Part model, mm, in its own coordinate system. Coordinates: 2 decimals unless noted, no trailing zeros. Loops run counter-clockwise (first coordinate to the right, second up) from the corner with the lowest first, then second, coordinate; pieces in that order, holes last. Notation, with made-up numbers: (52.25, 57) - (82.25, 57) arc R19 ccw to (82.25, 72) - close; hole circle Ø10 at (-14.75, 18.5). An arc over 180 degrees is marked (long way). Use a Markdown table: item, result. Add a question column.
1. Band-saw the part on C-C, the plane x = -0.75. Give the cut face in (y, z).
2. Drop flat-ended pins along their axis: pin 1 (1 mm diameter, centred on y = 124, z = 1.5, fed in from -X); pin 2 (1.5 mm diameter, centred on x = 1.5, y = 152, fed in from -Z); pin 3 (1 mm diameter, centred on y = 115.5, z = -2, fed in from -X). Give the stop position or say it passes through.
3. Band-saw the part on A-A, the plane y = 126.5. Give the cut face in (x, z).
4. Wall check: probe 1 along X at (y, z) = (113.5, -0.3); probe 2 along Z at (x, y) = (0.2, 130.5); probe 3 along X at (y, z) = (157.5, -0.5). Give the ranges that are in metal, low to high. Write a range as [from, to].
5. Band-saw the part on B-B, the plane z = 0.7. Give the cut face in (x, y).
from build123d import *

# Parameters (mm, degrees)
SKETCH_1_R               = 2.5
EXTRUDE_1_DEPTH          = 173.2
SKETCH_3_R               = 77
EXTRUDE_4_DEPTH          = 4
SKETCH_8_R               = 15
EXTRUDE_7_DEPTH          = 3
CUT_EXTRUDE_2_REACH      = 198.527
SKETCH_9_R               = 5
PATTERN_CIRCULAR_1_COUNT = 3
SKETCH_11_R              = 2.5
CUT_EXTRUDE_4_DEPTH      = 143.040275978
EXTRUDE_START            = 6.6
SKETCH_12_R              = 2.5
EXTRUDE_8_DEPTH          = 6.6
CUT_EXTRUDE_6_REACH      = 138.076
SKETCH_13_R              = 77
SKETCH_13_R_2            = 15
SKETCH_14_R              = 15
CUT_EXTRUDE_7_DEPTH      = 10
SKETCH_15_R              = 2.5
EXTRUDE_9_DEPTH          = 10


with BuildPart() as part:
    # Sketch 1 → Extrude 1 (new body)
    with BuildSketch(Plane(origin=(0, 0, 0), x_dir=(1, 0, 0), z_dir=(0, 1, 0))):
        with Locations(Location((0, 0, 0), (0, 0, 90))):
            Circle(SKETCH_1_R)
    extrude(amount=EXTRUDE_1_DEPTH)

    # Sketch 3 → Extrude 4 (add)
    with BuildSketch(Plane(origin=(0, 163.6, 0), x_dir=(1, 0, 0), z_dir=(0, 1, 0))):
        with Locations(Location((0, 0, 0), (0, 0, 270))):
            Circle(SKETCH_3_R)
    extrude(amount=-EXTRUDE_4_DEPTH)

    # Sketch 8 → Extrude 7 (add)
    with BuildSketch(Plane(origin=(0, 159.6, 0), x_dir=(-1, 0, 0), z_dir=(0, -1, 0))):
        with Locations(Location((0, 0, 0), (0, 0, 270))):
            Circle(SKETCH_8_R)
    extrude(amount=EXTRUDE_7_DEPTH)

    # Sketch 9 → Cut-Extrude 2 (cut, up to next)
    with BuildSketch(Plane(origin=(0, 163.6, 0), x_dir=(1, 0, 0), z_dir=(0, 1, 0)), mode=Mode.PRIVATE) as cut_extrude_2_sk1:
        with Locations(Location((0, 45, 0), (0, 0, 270))):
            Circle(SKETCH_9_R)
    cut_extrude_2_tool1 = extrude(cut_extrude_2_sk1.sketch, amount=-CUT_EXTRUDE_2_REACH, mode=Mode.PRIVATE) & part.part
    cut_extrude_2 = cut_extrude_2_tool1.solids().sort_by_distance((0, 163.6, -45))[0]
    add(cut_extrude_2, mode=Mode.SUBTRACT)

    # Pattern Circular 1: Cut-Extrude 2 ×3 about axis
    pattern_circular_1_axis = Axis((0, 0, 0), (0, 1, 0))
    for i in range(1, PATTERN_CIRCULAR_1_COUNT):
        add(cut_extrude_2.rotate(pattern_circular_1_axis, i * 360 / PATTERN_CIRCULAR_1_COUNT), mode=Mode.SUBTRACT)

    # Sketch 11 → Cut-Extrude 4 (cut, through all)
    with BuildSketch(Plane(origin=(0, 82, 0), x_dir=(1, 0, 0), z_dir=(0, 1, 0))):
        with Locations(Location((0, 0, 0), (0, 0, 90))):
            Circle(SKETCH_11_R)
    extrude(amount=-CUT_EXTRUDE_4_DEPTH, mode=Mode.SUBTRACT)

    # Sketch 12 → Extrude 8 (add)
    with BuildSketch(Plane(origin=(0, 153.6, 0), x_dir=(-1, 0, 0), z_dir=(0, -1, 0)).offset(EXTRUDE_START)):
        with Locations(Location((0, 0, 0), (0, 0, 90))):
            Circle(SKETCH_12_R)
    extrude(amount=-EXTRUDE_8_DEPTH)

    # Sketch 13 → Cut-Extrude 6 (cut, up to next)
    with BuildSketch(Plane(origin=(0, 163.6, 0), x_dir=(1, 0, 0), z_dir=(0, 1, 0)), mode=Mode.PRIVATE) as cut_extrude_6_sk1:
        Circle(SKETCH_13_R)
        with Locations(Location((0, 0, 0), (0, 0, 270))):
            Circle(SKETCH_13_R_2, mode=Mode.SUBTRACT)
    cut_extrude_6_tool1 = extrude(cut_extrude_6_sk1.sketch, amount=-CUT_EXTRUDE_6_REACH, mode=Mode.PRIVATE) & part.part
    add(cut_extrude_6_tool1.solids().sort_by_distance((-74.822111, 163.6, 0))[0], mode=Mode.SUBTRACT)

    # Sketch 14 → Cut-Extrude 7 (cut)
    with BuildSketch(Plane(origin=(0, 163.6, 0), x_dir=(1, 0, 0), z_dir=(0, 1, 0))):
        Circle(SKETCH_14_R)
    extrude(amount=-CUT_EXTRUDE_7_DEPTH, mode=Mode.SUBTRACT)


with BuildPart() as cut_extrude_7_piece_1:
    # of the separate pieces the step leaves, piece 1, a body of its own (cut_extrude_7_pieces)
    add(part.part.solids().sort_by_distance((0, 82, -2.5))[0])



with BuildPart() as cut_extrude_7_piece_2:
    # of the separate pieces the step leaves, piece 2, a body of its own (cut_extrude_7_pieces)
    add(part.part.solids().sort_by_distance((0, 163.6, -2.5))[0])


with BuildPart() as cut_extrude_7_piece_1_1:
    add(cut_extrude_7_piece_1.part)

    add(cut_extrude_7_piece_2.part)  # Extrude 9 merges Cut-Extrude 7 piece 2
    # Sketch 15 → Extrude 9 (add)
    with BuildSketch(Plane(origin=(0, 153.6, 0), x_dir=(-1, 0, 0), z_dir=(0, -1, 0))):
        with Locations(Location((0, 0, 0), (0, 0, 90))):
            Circle(SKETCH_15_R)
    extrude(amount=-EXTRUDE_9_DEPTH)


solid = cut_extrude_7_piece_1_1.part
Geometry check:
| question | item | result |
|---|---|---|
| 1 | outline | (82, -2.38) - (173.2, -2.38) - (173.2, 2.38) - (82, 2.38) - close |
| 2 | pin 1 | stops at x = -2.29 |
| 2 | pin 2 | stops at z = -2.38 |
| 2 | pin 3 | stops at x = -2 |
| 3 | outline | circle Ø5 at (0, 0) |
| 4 | probe 1 | x = [-2.48, 2.48] |
| 4 | probe 2 | z = [-2.49, 2.49] |
| 4 | probe 3 | x = [-2.45, 2.45] |
| 5 | outline | (-2.4, 82) - (2.4, 82) - (2.4, 173.2) - (-2.4, 173.2) - close |
